from build123d import *

# Parameters (mm, degrees)
SKETCH1_W           = 125
SKETCH1_H           = 30
SKETCH1_R           = 7.5
BOSS_EXTRUDE1_DEPTH = 10
SKETCH3_W           = 125
SKETCH3_H           = 20
BOSS_EXTRUDE2_DEPTH = 10
SKETCH4_R           = 7.5
BOSS_EXTRUDE3_DEPTH = 40


with BuildPart() as part:
    # Sketch1 → Boss-Extrude1 (new body)
    with BuildSketch(Plane(origin=(0, 0, 0), x_dir=(1, 0, 0), z_dir=(0, 1, 0))):
        Rectangle(SKETCH1_W, SKETCH1_H)
        with Locations(Location((-45, 0, 0), (0, 0, 270))):
            Circle(SKETCH1_R, mode=Mode.SUBTRACT)
        with Locations(Location((45, 0, 0), (0, 0, 270))):
            Circle(SKETCH1_R, mode=Mode.SUBTRACT)
    extrude(amount=BOSS_EXTRUDE1_DEPTH)

    # Sketch3 → Boss-Extrude2 (add)
    with BuildSketch(Plane.XZ):
        Rectangle(SKETCH3_W, SKETCH3_H)
    extrude(amount=BOSS_EXTRUDE2_DEPTH)

    # Sketch4 → Boss-Extrude3 (add)
    with BuildSketch(Plane(origin=(0, 0, 0), x_dir=(1, 0, 0), z_dir=(0, 1, 0))):
        with Locations(Location((45, 0, 0), (0, 0, 270))):
            Circle(SKETCH4_R)
        with Locations(Location((-45, 0, 0), (0, 0, 270))):
            Circle(SKETCH4_R)
    extrude(amount=BOSS_EXTRUDE3_DEPTH)


solid = part.part
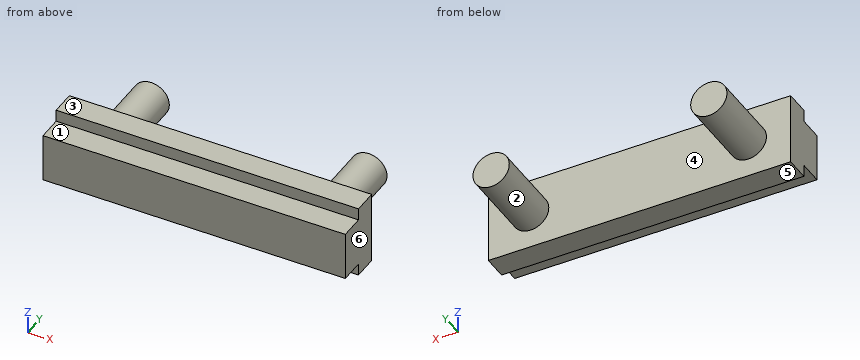
Work out the finished part from the listing and answer in its coordinate system (mm). Face numbers are marked on the shaded views. A direction names the side the tool comes from. Give positions to 0.01 mm unless a question says otherwise; leave off trailing zeros. Loops run counter-clockwise (first coordinate to the right, second up) from the corner with the lowest first, then second, coordinate; pieces in that order, holes last. Notation, with made-up numbers: (53.25, -35.75) -> (66.25, -35.75) arc R14 ccw to (66.25, -25.75) -> close; hole circle Ø9 at (-2.75, 33). An arc over 180 degrees is marked (long way). Use a Markdown table: item, result. Add a question column.
1) The part is cut by section A-A, the plane y = 17.5. Determine the outline of the cut face in (x, z).
2) For a pull along X with two mould halves and no side action, classify the marked faces 4, 5 and 6 as +X half, -X half, draft (parallel to the pull), parting line (faces both ways), or undercut.
3) Which of the six approach directions +Z, -Z, +X, -X, +Y, -Y give full straight-line access (tool end or side, diameter ignored) to the marked faces 1, 2 and 3?
4) The part is cut by section B-B, the plane x = -24. Determine the outline of the cut face in (y, z).
5) The part is cut by section D-D, the plane y = -6. Determine the outline of the cut face in (x, z), plus the area to 3 significant figures.
6) The part is cut by section C-C, the plane z = 0. Determine the outline of the cut face in (x, y), plus the area to 3 significant figures.
7) Each of these flat-tipped pins is pushed along its axis until it touches: P1, Ø8, axis at y = 33.5, z = -1.5, coming from the +X side; P2, Ø1.5, axis at y = 14, z = -4.5, coming from the +X side; P3, Ø5, axis at x = -22, y = -5, coming from the +Z side. Where does it stop, or does it pass through?
8) Consider line 1 along X through (y, z) = (19, -0.5); line 2 along Y through (x, z) = (-29, 5.25); line 3 along Y through (x, z) = (-51, 12.75). Determine where each line is inside the solid, lowest interval first.
Reported:
| question | item | result |
|---|---|---|
| 1 | outline | circle Ø15 at (-45, 0); circle Ø15 at (45, 0) |
| 2 | face 4 | undercut |
| 2 | face 5 | draft |
| 2 | face 6 | +X half |
| 3 | face 1 | +Z, +X, -X, -Y |
| 3 | face 2 | +Y |
| 3 | face 3 | +Z, +X, -X, +Y, -Y |
| 4 | outline | (-10, -10) -> (0, -10) -> (0, -15) -> (10, -15) -> (10, 15) -> (0, 15) -> (0, 10) -> (-10, 10) -> close |
| 5 | outline | (-62.5, -10) -> (62.5, -10) -> (62.5, 10) -> (-62.5, 10) -> close |
| 5 | area | 2,500 mm^2 |
| 6 | outline | (-62.5, -10) -> (62.5, -10) -> (62.5, 10) -> (52.5, 10) -> (52.5, 40) -> (37.5, 40) -> (37.5, 10) -> (-37.5, 10) -> (-37.5, 40) -> (-52.5, 40) -> (-52.5, 10) -> (-62.5, 10) -> close |
| 6 | area | 3,400 mm^2 |
| 7 | P1 | stops at x = 52.5 |
| 7 | P2 | stops at x = 51.5 |
| 7 | P3 | stops at z = 10 |
| 8 | line 1 | x = -52.48 to -37.52, 37.52 to 52.48 |
| 8 | line 2 | y = -10 to 10 |
| 8 | line 3 | y = 0 to 10 |
